Work out the finished part from the listing and answer in its coordinate system (mm). Face numbers are marked on the shaded views. A direction names the side the tool comes from. Round coordinates to 2 decimals unless told otherwise and drop trailing zeros. Order: outer loops, then holes, each group sorted by start corner. A loop starts at its lowest first (then second) coordinate and runs counter-clockwise, first axis right, second up. Notation, with made-up numbers: M 81.5,-3.5 L 98.5,-3.5 A19 ccw 98.5,30.5 Z; hole C 80.5,43 d5. An arc over 180 degrees is marked long. Return JSON: item names as keys, results as strings.
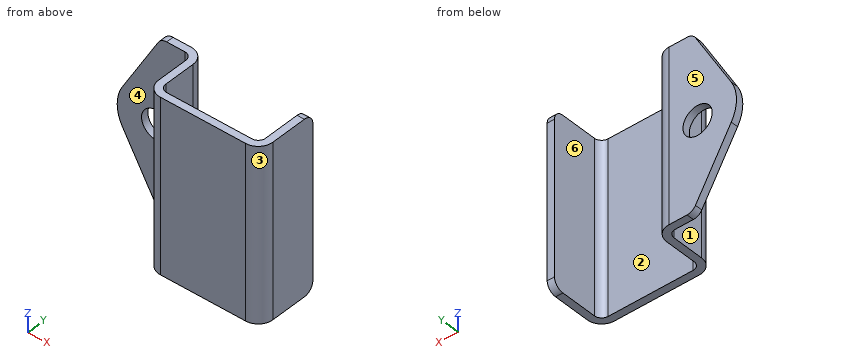
Autodesk Inventor part; units mm, degrees
ref_plane "YZ Plane" through (0, 0, 0) normal (1, 0, 0) x (0, 1, 0)
ref_plane "XZ Plane" through (0, 0, 0) normal (0, 1, 0) x (-1, 0, 0)
ref_plane "XY Plane" through (0, 0, 0) normal (0, 0, 1) x (1, 0, 0)
sketch "Sketch1" plane through (0, 0, 0) normal (0, 1, 0) x (-1, 0, 0)
  line L0 (-20.5, 35.5) -> (20.5, 35.5)
  line L1 (20.5, 35.5) -> (20.5, -35.5)
  line L2 (20.5, -35.5) -> (-20.5, -35.5)
  line L3 (-20.5, -35.5) -> (-20.5, 35.5)
  line L4 (-20.5, 35.5) -> (20.5, -35.5) construction
  line L5 (20.5, 35.5) -> (-20.5, -35.5) construction
  point P0 (0, 0)
  point P1 (0, 0)
  point P2 (0, 0)
  dimension "d0" = 71
  dimension "d1" = 41
extrude "Plate1" add sketch "Sketch1" along normal blind 3
sketch "Sketch2" plane through (20.5, 3, -35.5) normal (1, 0, 0) x (0, 1, 0)
  line L0 (0, 71) -> (0, 0)
  line L1 (0, 0) -> (22, 0)
  line L2 (22, 0) -> (22, 71)
  line L3 (22, 71) -> (0, 71)
edge flange "Flange1" height 22 angle 90 thickness 3 bend radius 3 thickness toward (1, 0, 0) relief tear relief width 3 relief depth 1.5 corner gap 3 corner form 0 edges at (20.5, 3, 0) (-20.5, 3, 0) wall of the first edge with corners at (20.5, 3, 35.5) (20.5, 3, -35.5) (20.5, 25, -35.5) (20.5, 25, 35.5)
bend "Bend1"
corner "Corner1"
sketch "Sketch3" plane through (-20.5, 22, -35.5) normal (0, 1, 0) x (-1, 0, 0)
  line L0 (0, 71) -> (0, 0)
  line L1 (0, 0) -> (33.8, 0)
  line L2 (33.8, 0) -> (33.8, 71)
  line L3 (33.8, 71) -> (0, 71)
edge flange "Flange2" height 33.8 angle 90 thickness 3 bend radius 3 thickness toward (0, 1, 0) relief tear relief width 3 relief depth 1.5 edges at (-23.5, 25, 0) wall of the first edge with corners at (-20.5, 22, 35.5) (-20.5, 22, -35.5) (-54.3, 22, -35.5) (-54.3, 22, 35.5)
bend "Bend2"
corner "Corner2"
sketch "Sketch4" plane through (-54.3, 25, 35.5) normal (0, 1, 0) x (1, 0, 0)
  line L0 (0, 0) -> (28.3, 0)
  line L1 (28.3, 71) -> (0, 71)
  line L2 (0, 0) -> (0, 71)
  line L3 (54.3, 35.5) -> (0, 35.5) construction
  line L4 (2.1436, 27.5) -> (18.0207, 0)
  line L5 (2.1436, 43.5) -> (18.0207, 71)
  arc A0 (2.1436, 43.5) -> (2.1436, 27.5) centre (16, 35.5) ccw
  line L6 (74.8, 71) -> (77.8, 71)
  line L7 (74.8, 0) -> (77.8, 0)
  point P0 (54.3, 35.5)
  dimension "d23" = 30
  dimension "d24" = 30
  dimension "d25" = 16
  dimension "d26" = 38.3
extrude "Cut1" cut sketch "Sketch4" against normal blind 3
fillet "Fillet1" radius 4 4 edges at (-36.2793, 23.5, 35.5) (-36.2793, 23.5, -35.5) (22, 25, -35.5) (22, 25, 35.5)
sketch "Sketch5" plane through (-26.5, 25, 35.5) normal (0, 1, 0) x (1, 0, 0)
  arc A0 (-25.6564, 43.5) -> (-25.6564, 27.5) centre (-11.8, 35.5) ccw
  circle A1 centre (-11.8, 35.5) radius 6
  point P0 (26.5, 35.5)
  dimension "d30" = 12
extrude "Extrusion1" cut sketch "Sketch5" against normal through all
equation "\"d24\" = d23"
equation "\"d27\" = Thickness"
equation "\"d2\" = Thickness"
equation "\"d3\" = BendReliefWidth"
equation "\"d4\" = BendReliefDepth"
equation "\"d5\" = MinimumRemnant"
equation "\"d6\" = TransitionRadius"
equation "\"d9\" = BendRadius"
equation "\"d10\" = CornerReliefSize"
equation "\"d11\" = GapSize"
equation "\"d12\" = JacobiRadiusSize"
equation "\"d13\" = BendReliefWidth"
equation "\"d14\" = BendReliefDepth"
equation "\"d15\" = MinimumRemnant"
equation "\"d16\" = TransitionRadius"
equation "\"d19\" = BendRadius"
equation "\"d20\" = CornerReliefSize"
equation "\"d21\" = GapSize"
equation "\"d22\" = JacobiRadiusSize"
equation "\"BendRadius\" = Thickness"
equation "\"BendReliefWidth\" = Thickness"
equation "\"BendReliefDepth\" = 0.5 * Thickness"
equation "\"CornerReliefSize\" = 4 * Thickness"
equation "\"MinimumRemnant\" = 2 * Thickness"
equation "\"TransitionRadius\" = BendRadius"
equation "\"JacobiRadiusSize\" = BendRadius"
equation "\"GapSize\" = Thickness"
properties part number "318-02" material "Aluminum 6061"
Item 1: Find section B-B (z = 0). Determine the outline of the cut face in (x, y), plus the area to 3 significant figures.
Output:
{"outline": "M -54.3,22 L -44.3,22 L -44.3,25 L -54.3,25 Z; M -32.3,22 L -26.5,22 A3 cw -23.5,19 L -23.5,6 A6 ccw -17.5,0 L 17.5,0 A6 ccw 23.5,6 L 23.5,25 L 20.5,25 L 20.5,6 A3 cw 17.5,3 L -17.5,3 A3 cw -20.5,6 L -20.5,19 A6 ccw -26.5,25 L -32.3,25 Z", "area": "312 mm^2"}
Item 2: Which of the six approach directions +Z, -Z, +X, -X, +Y, -Y give full straight-line access (tool end or side, diameter ignored) to the marked faces 4, 5 and 6?
Output:
{"face 4": "+Z, -Z, -X, -Y", "face 5": "+Z, -Z, +X, -X, +Y", "face 6": "+Z, -Z, +Y"}
Item 3: Find section D-D (y = 23.75). Determine the outline of the cut face in (x, z), plus the area to 3 significant figures.
Output:
{"outline": "M -52.16,-8 L -37.43,-33.5 A4 ccw -33.97,-35.5 L -22.83,-35.5 L -22.83,35.5 L -33.97,35.5 A4 ccw -37.43,33.5 L -52.16,8 A16 ccw Z; M 20.5,-34.4 L 23.5,-34.4 L 23.5,34.4 L 20.5,34.4 Z; hole C -38.3,0 d12", "area": "1,760 mm^2"}
Item 4: The mould has two halves that part along X. Classify the marked faces 1, 2 and 3: pulls with the +X half, pulls with the -X half, needs draft (parallel to the pull), parting line crosses it, or undercut.
Output:
{"face 1": "pulls with the -X half", "face 2": "undercut", "face 3": "pulls with the +X half"}
Item 5: Find section A-A (y = 10.5). Determine the outline of the cut face in (x, z).
Output:
{"outline": "M -23.5,-35.5 L -20.5,-35.5 L -20.5,35.5 L -23.5,35.5 Z; M 20.5,-35.5 L 23.5,-35.5 L 23.5,35.5 L 20.5,35.5 Z"}
Item 6: Find section C-C (x = -38.5). Determine the outline of the cut face in (y, z).
Output:
{"outline": "M 22,-31.65 L 25,-31.65 L 25,-6 L 22,-6 Z; M 22,6 L 25,6 L 25,31.65 L 22,31.65 Z"}
Item 7: Each of these flat-tipped pins is pushed along its axis until it touches: pin 1 (3 mm diameter, centred on x = -41.5, z = 27.5, fed in from +Y); pin 2 (5 mm diameter, centred on y = 21, z = -15, fed in from -X); pin 3 (14 mm diameter, centred on x = -34.5, z = 7.5, fed in from -Y); pin 4 (10.5 mm diameter, centred on y = 12, z = 0.5, fed in from -X). Where does it stop, or does it pass through?
Output:
{"pin 1": "stops at y = 25", "pin 2": "stops at x = -49.44", "pin 3": "stops at y = 22", "pin 4": "stops at x = -23.5"}
Item 8: Consider line 1 along X through (y, z) = (24.2, 0); line 2 along X through (y, z) = (16, 22.5); line 3 along X through (y, z) = (23.75, 0). Determine where each line is inside the solid, lowest interval first. Write a range as [from, to].
Output:
{"line 1": "x = [-54.3, -44.3], [-32.3, -23.51], [20.5, 23.5]", "line 2": "x = [-23.5, -20.5], [20.5, 23.5]", "line 3": "x = [-54.3, -44.3], [-32.3, -22.83], [20.5, 23.5]"}
